```python
from build123d import *

# Parameters (mm, degrees)
PAD_DEPTH = 20


with BuildPart() as part:
    # Sketch → Pad (new body)
    with BuildSketch(Plane.XZ):
        Polygon((3.95, 8.4), (3.95, 1), (4.95, 1), (4.95, 0), (0, 0), (0, 1), (2.65, 1), (2.65, 7.4), (0, 7.4), (0, 8.4), align=None)
    pad = extrude(amount=PAD_DEPTH)

    # Mirrored: Pad across Sketch V_Axis
    add(pad.mirror(Plane(origin=(0, 0, 0), x_dir=(0, -1, 0), z_dir=(1, 0, 0))))


solid = part.part
```
Geometry: final body of the model. Coordinates: model frame, mm. A direction names the side the tool comes from. Round coordinates to 2 decimals unless told otherwise and drop trailing zeros. Loops run counter-clockwise (first coordinate to the right, second up) from the corner with the lowest first, then second, coordinate; pieces in that order, holes last.
Item 1: Section C-C, the plane y = -1.75. Output: boundary loops of the cut face in (x, z).
Checked values:
outline: (-4.95, 0) - (4.95, 0) - (4.95, 1) - (3.95, 1) - (3.95, 8.4) - (-3.95, 8.4) - (-3.95, 1) - (-4.95, 1) - close; hole (-2.65, 1) - (2.65, 1) - (2.65, 7.4) - (-2.65, 7.4) - close
Item 2: Mould query, pull axis X, two halves, no side actions, for faces 1 (the flat face through (4.4, -9.9, 1)), 2 (the flat face through (2.65, -10, 4)), 3 (the flat face through (-2.65, -10, 4)), 4 (the flat face through (4.95, -9.9, 0.5)). Classes: released by +X, released by -X, zero draft, split by the parting line, or undercut.
Checked values:
face 1: zero draft
face 2: undercut
face 3: undercut
face 4: released by +X
Item 3: Contact query for flat-ended pins moving along their axis: P1, Ø1.9, axis at y = -6.5, z = 4, coming from the -X side; P2, Ø0.8, axis at x = -4.5, y = -8, coming from the +Z side; P3, Ø3.5, axis at y = -11.5, z = 4, coming from the +X side. Output: stop coordinate, or through.
Checked values:
P1: stops at x = -3.95
P2: stops at z = 1
P3: stops at x = 3.95
Item 4: Section B-B, the plane z = 2. Output: boundary loops of the cut face in (x, y), plus the area to 3 significant figures.
Checked values:
outline: (-3.95, -20) - (-2.65, -20) - (-2.65, 0) - (-3.95, 0) - close; (2.65, -20) - (3.95, -20) - (3.95, 0) - (2.65, 0) - close
area: 52.0 mm2
Item 5: Line query: L1, parallel to X at y = -0.75, z = 5; L2, parallel to Z at x = 1.75, y = -6.5; L3, parallel to Z at x = 4.5, y = -2.5. Output: solid intervals per line, ascending.
Checked values:
L1: x = -3.95 to -2.65, 2.65 to 3.95
L2: z = 0 to 1, 7.4 to 8.4
L3: z = 0 to 1
Item 6: Reachability of faces 5 (the flat face through (-4.95, -9.9, 0.5)), 6 (the flat face through (-3.95, -10, 5)), 7 (the flat face through (0, -10, 0)), 8 (the flat face through (0, -10, 7.4)), 9 (the flat face through (3.95, -10, 5)) from +Z, -Z, +X, -X, +Y, -Y: full face, straight path, thin tool, end or side. Return the list, or none.
Checked values:
face 5: +Z, -Z, -X, +Y, -Y
face 6: +Z, -X, +Y, -Y
face 7: -Z, +X, -X, +Y, -Y
face 8: +Y, -Y
face 9: +Z, +X, +Y, -Y
Item 7: Section D-D, the plane x = 4.25. Output: boundary loops of the cut face in (y, z), plus the area to 3 significant figures.
Checked values:
outline: (-20, 0) - (0, 0) - (0, 1) - (-20, 1) - close
area: 20.0 mm2
Item 8: Section A-A, the plane x = 0.75. Output: boundary loops of the cut face in (y, z), plus the area to 3 significant figures.
Checked values:
outline: (-20, 0) - (0, 0) - (0, 1) - (-20, 1) - close; (-20, 7.4) - (0, 7.4) - (0, 8.4) - (-20, 8.4) - close
area: 40.0 mm2
